```python
from build123d import *

# Parameters (mm, degrees)
CROQUIS2_R              = 1.5
CROQUIS2_R_2            = 1
CROQUIS2_R_3            = 3.75
SALIENTE_EXTRUIR1_DEPTH = 3


with BuildPart() as part:
    # Croquis2 → Saliente-Extruir1 (new body)
    with BuildSketch(Plane.XY):
        with BuildLine():
            Line((10, 0), (10, 30))
            add(Edge.make_bspline(
                [(10, 40), (13.382456464, 40), (10, 31.604422757), (10, 30)],
                knots=[0, 0, 0, 0, 1, 1, 1, 1], degree=3))
            ThreePointArc((10, 40), (7.878679656, 40.878679656), (7, 43))
            Line((7, 43), (7, 50))
            Line((7, 50), (5, 50))
            Line((5, 50), (5, 45))
            ThreePointArc((5, 45), (3.535533906, 41.464466094), (0, 40))
            ThreePointArc((0, 40), (-1.767766953, 39.267766953), (-2.5, 37.5))
            Line((-2.5, 37.5), (-2.5, 37.3))
            ThreePointArc((-2.5, 37.3), (-3.173654403, 35.673654403), (-4.8, 35))
            Line((-4.8, 35), (-5, 35))
            ThreePointArc((-5, 35), (-5.707106781, 34.707106781), (-6, 34))
            Line((-6, 34), (-6, 30))
            Line((-6, 30), (-6, 16.38315603))
            ThreePointArc((-6, 16.38315603), (-6.292893219, 15.676049249), (-7, 15.38315603))
            Line((-7, 15.38315603), (-9, 15.38315603))
            ThreePointArc((-9, 15.38315603), (-9.707106781, 15.090262811), (-10, 14.38315603))
            Line((-10, 14.38315603), (-10, 0))
            Line((-10, 0), (10, 0))
        make_face()
        with Locations((0, 37.5)):
            Circle(CROQUIS2_R, mode=Mode.SUBTRACT)
        with Locations((0, 33)):
            Circle(CROQUIS2_R_2, mode=Mode.SUBTRACT)
        with Locations((0, 4)):
            Circle(CROQUIS2_R_2, mode=Mode.SUBTRACT)
        with Locations((0, 24)):
            Circle(CROQUIS2_R_3, mode=Mode.SUBTRACT)
    extrude(amount=SALIENTE_EXTRUIR1_DEPTH)


solid = part.part
```
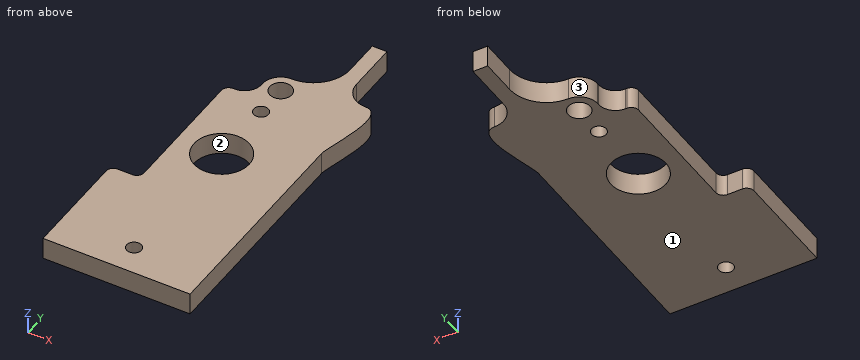
Source: CAD feature listing. Evaluate the final solid. Frame: model axes, mm. Face numbers are marked on the shaded views. Coordinates: 2 decimals unless noted, no trailing zeros. Loops run counter-clockwise (first coordinate to the right, second up) from the corner with the lowest first, then second, coordinate; pieces in that order, holes last. Notation, with made-up numbers: M 47,-37.75 L 76,-37.75 A12 ccw 76,-31.75 Z; hole C 42.25,72 d5. An arc over 180 degrees is marked long. Use CSV: the item, a comma, the result in double quotes.
(1) Cut plane C-C on x = 0.5. Return loops of the section in (y, z).
Answers follow:
outline,"M 0,0 L 3.13,0 L 3.13,3 L 0,3 Z; M 4.87,0 L 20.28,0 L 20.28,3 L 4.87,3 Z; M 27.72,0 L 32.13,0 L 32.13,3 L 27.72,3 Z; M 33.87,0 L 36.09,0 L 36.09,3 L 33.87,3 Z; M 38.91,0 L 40.03,0 L 40.03,3 L 38.91,3 Z"
(2) Draft query along Y for the marked faces 1, 2 and 3. Return one class per face: pulls with the +Y half, pulls with the -Y half, needs draft (parallel to the pull), parting line crosses it, or undercut.
Answers follow:
face 1,"needs draft"
face 2,"undercut"
face 3,"pulls with the +Y half"
(3) Line query: line 1 (Y direction, x = 0, z = 1.9); line 2 (Y direction, x = 1.25, z = 0.35); line 3 (Y direction, x = -7, z = 1.1). Output: solid intervals per line, ascending. Write a range as [from, to].
Answers follow:
line 1,"[0, 3], [5, 20.25], [27.75, 32], [34, 36], [39, 40]"
line 2,"[0, 20.46], [27.54, 36.67], [38.33, 40.16]"
line 3,"[0, 15.38]"
(4) Cut plane B-B on y = 4. Return loops of the section in (x, z).
Answers follow:
outline,"M -10,0 L -1,0 L -1,3 L -10,3 Z; M 1,0 L 10,0 L 10,3 L 1,3 Z"
(5) Cut plane D-D on z = 1.75. Give the number of separate pieces and of enclosed holes in the cut face, and give its area (3 significant figures).
Answers follow:
separate pieces,"1"
enclosed holes,"4"
area,"663 mm²"
(6) Contact query for flat-ended pins moving along their axis: pin 1 (1.5 mm diameter, centred on y = 38, z = 1, fed in from -X); pin 2 (1 mm diameter, centred on x = -8, z = 2, fed in from +Y); pin 3 (0.9 mm diameter, centred on y = 46, z = 1.5, fed in from +X). Output: stop coordinate, or through.
Answers follow:
pin 1,"x = -2.5"
pin 2,"y = 15.38"
pin 3,"x = 7"
(7) Cut plane A-A on x = 3. Return loops of the section in (y, z).
Answers follow:
outline,"M 0,0 L 21.75,0 L 21.75,3 L 0,3 Z; M 26.25,0 L 41,0 L 41,3 L 26.25,3 Z"
